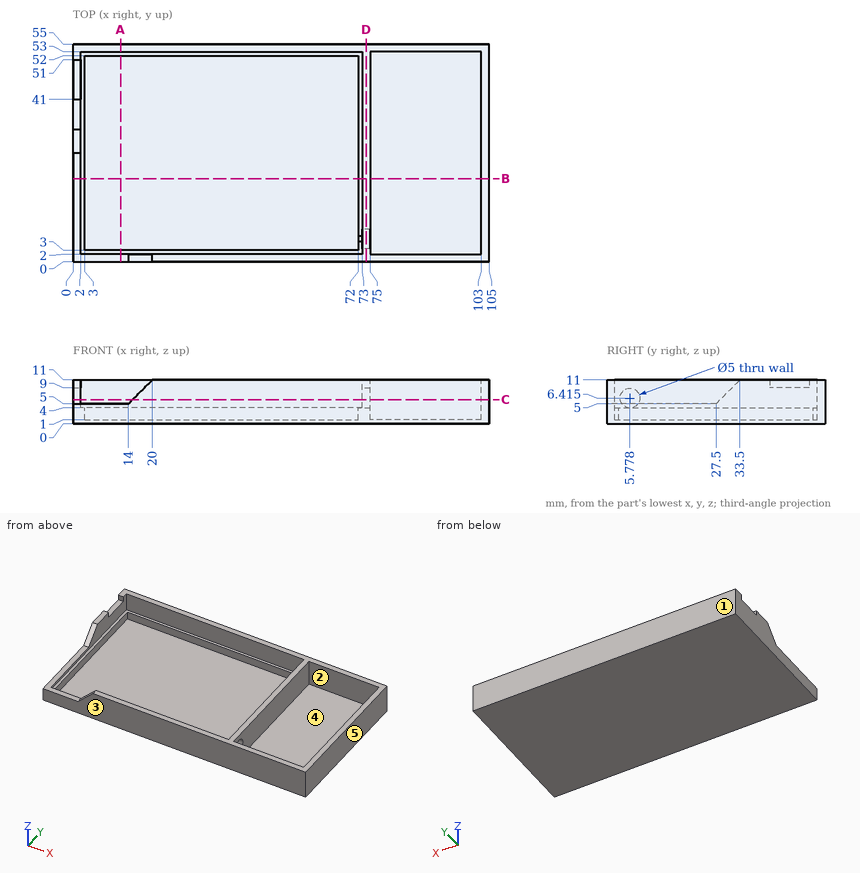
Check sheet for the drawn part. Datum: minimum x, y, z corner. Units: mm. A direction names the side the tool comes from. Round coordinates to 2 decimals unless told otherwise and drop trailing zeros. Order: outer loops, then holes, each group sorted by start corner. A loop starts at its lowest first (then second) coordinate and runs counter-clockwise, first axis right, second up.
1) Section check B-B (y = 21). Record the boundary of the cut face in (x, z), and give its area (3 significant figures).
2) Mould release check, pull along X, two halves, no side actions. Record for the marked faces 3, 4 and 5: +X half, -X half, draft (parallel to the pull), parting line (faces both ways), or undercut.
3) Section check D-D (x = 74). Record the boundary of the cut face in (y, z) (1 decimal), and give its area (3 significant figures).
4) Go/stop test with flat-tipped pins: pin 1 Ø0.9 at (x, z) = (30.5, 2) entering from -Y; pin 2 Ø14 at (x, y) = (88, 20.5) entering from +Z; pin 3 Ø1 at (y, z) = (13, 8.5) entering from -X; pin 4 Ø1 at (x, z) = (0.5, 9.5) entering from -Y. Record where each tip stops, or that it passes through.
5) Section check C-C (z = 6). Record the boundary of the cut face in (x, y).
6) Section check A-A (x = 12). Record the boundary of the cut face in (y, z).
7) Scan lines: line 1 (X direction, y = 40, z = 3.25); line 2 (X direction, y = 40.5, z = 10); line 3 (X direction, y = 43, z = 9.75). Record each from-to range of solid material in increasing order.
8) Tool access check on the marked faces 1 and 2. Record the directions out of +Z, -Z, +X, -X, +Y, -Y that give a thin tool (end or side, any length) a straight path to the whole face; none if there is none.
Result:
1. outline: (0, 0) - (105, 0) - (105, 11) - (103, 11) - (103, 1) - (75, 1) - (75, 11) - (73, 11) - (73, 4) - (72, 4) - (72, 1) - (3, 1) - (3, 4) - (2, 4) - (2, 5) - (0, 5) - close
1. area: 159 mm2
2. face 3: draft
2. face 4: undercut
2. face 5: +X half
3. outline: (0, 0) - (55, 0) - (55, 11) - (0, 11) - close; hole circle Ø5 at (5.8, 6.4)
3. area: 585 mm2
4. pin 1: stops at y = 0
4. pin 2: stops at z = 1
4. pin 3: stops at x = 73
4. pin 4: stops at y = 31.5
5. outline: (0, 28.5) - (2, 28.5) - (2, 53) - (73, 53) - (73, 8.24) - (75, 8.24) - (75, 53) - (103, 53) - (103, 2) - (75, 2) - (75, 3.31) - (73, 3.31) - (73, 2) - (15, 2) - (15, 0) - (105, 0) - (105, 55) - (0, 55) - close
6. outline: (0, 0) - (55, 0) - (55, 11) - (53, 11) - (53, 4) - (52, 4) - (52, 1) - (3, 1) - (3, 4) - (2, 4) - (2, 5) - (0, 5) - close
7. line 1: x = 0 to 3, 72 to 75, 103 to 105
7. line 2: x = 0 to 2, 73 to 75, 103 to 105
7. line 3: x = 73 to 75, 103 to 105
8. face 1: +Z, -Z, +X, -X, +Y
8. face 2: +Z
